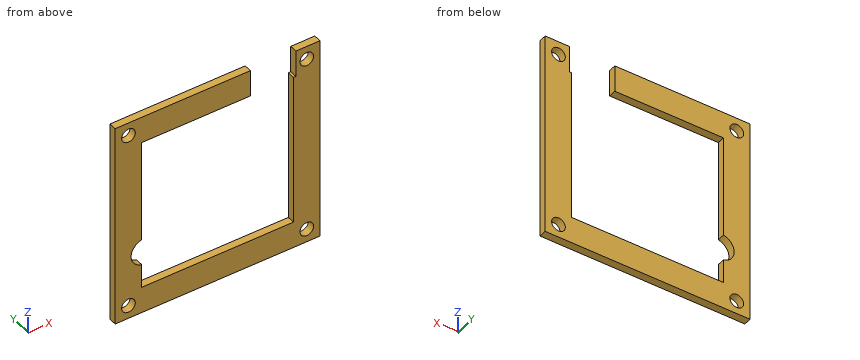
from build123d import *

# Parameters (mm, degrees)
SKETCH_3_R      = 1.8
EXTRUDE_2_DEPTH = 2


with BuildPart() as part:
    # 草图3 → 凸台-拉伸2 (new body)
    with BuildSketch(Plane(origin=(0, 0, 0), x_dir=(1, 0, 0), z_dir=(0, 1, 0))):
        with BuildLine():
            Line((20, 20), (20, -20))
            Line((20, -20), (20.65, -20))
            Line((20.65, -20), (20.65, -27))
            Line((20.65, -27), (27, -27))
            Line((27, -27), (27, 27))
            Line((27, 27), (-27, 27))
            Line((-27, 27), (-27, -27))
            Line((-27, -27), (8.65, -27))
            Line((8.65, -27), (8.65, -20))
            Line((8.65, -20), (-20, -20))
            Line((-20, -20), (-20, 6.87071436))
            ThreePointArc((-20, 6.87071436), (-22.8, 10.3), (-20, 13.72928564))
            Line((-20, 13.72928564), (-20, 20))
            Line((-20, 20), (-16.7, 20))
            Line((-16.7, 20), (-10.4, 20))
            Line((-10.4, 20), (-4.1, 20))
            Line((-4.1, 20), (20, 20))
        make_face()
        with Locations((-23.5, -23.5)):
            Circle(SKETCH_3_R, mode=Mode.SUBTRACT)
        with Locations((23.5, -23.5)):
            Circle(SKETCH_3_R, mode=Mode.SUBTRACT)
        with Locations((-23.5, 23.5)):
            Circle(SKETCH_3_R, mode=Mode.SUBTRACT)
        with Locations((23.5, 23.5)):
            Circle(SKETCH_3_R, mode=Mode.SUBTRACT)
    extrude(amount=EXTRUDE_2_DEPTH)


solid = part.part
Work out the finished part from the listing and answer in its coordinate system (mm). Round coordinates to 2 decimals unless told otherwise and drop trailing zeros. Loops run counter-clockwise (first coordinate to the right, second up) from the corner with the lowest first, then second, coordinate; pieces in that order, holes last. Notation, with made-up numbers: (-14, 54) - (29, 54) arc R13 cw to (29, 71) - close; hole circle Ø9 at (-8, 7). An arc over 180 degrees is marked (long way). One line per item, written item: value.
Q1. Find section B-B on x = 23.5. Give the vertices of the cut face in (y, z).
Check values:
outline: (0, -27) - (2, -27) - (2, -25.3) - (0, -25.3) - close; (0, -21.7) - (2, -21.7) - (2, 21.7) - (0, 21.7) - close; (0, 25.3) - (2, 25.3) - (2, 27) - (0, 27) - close
Q2. Each of these flat-tipped pins is pushed along its axis until it touches: pin 1 Ø0.7 at (x, y) = (20, 0.5) entering from +Z; pin 2 Ø4 at (x, z) = (-23.5, 23.5) entering from +Y; pin 3 Ø3 at (x, z) = (23.5, -23.5) entering from +Y. Where does it stop, or does it pass through?
Check values:
pin 1: z = 20
pin 2: y = 2
pin 3: through
Q3. Find section A-A on z = 6.5. Give the vertices of the cut face in (x, y).
Check values:
outline: (-27, 0) - (-20, 0) - (-20, 2) - (-27, 2) - close; (20, 0) - (27, 0) - (27, 2) - (20, 2) - close
Q4. Straight lines are drawn through the part: probe 1 along X at (y, z) = (0.55, -23.5); probe 2 along X at (y, z) = (1.6, 23.5). For each, find the intervals that lie inside material, in ascending order.
Check values:
probe 1: -27 to -25.3, -21.7 to 21.7, 25.3 to 27
probe 2: -27 to -25.3, -21.7 to 8.65, 20.65 to 21.7, 25.3 to 27
Q5. Find section C-C on y = 0.6. Give the vertices of the cut face in (x, z).
Check values:
outline: (-27, -27) - (27, -27) - (27, 27) - (20.65, 27) - (20.65, 20) - (20, 20) - (20, -20) - (-20, -20) - (-20, -13.73) arc R3.5 cw to (-20, -6.87) - (-20, 20) - (8.65, 20) - (8.65, 27) - (-27, 27) - close; hole circle Ø3.6 at (-23.5, -23.5); hole circle Ø3.6 at (-23.5, 23.5); hole circle Ø3.6 at (23.5, -23.5); hole circle Ø3.6 at (23.5, 23.5)
Q6. Find section D-D on z = 23.5. Give the vertices of the cut face in (x, y).
Check values:
outline: (-27, 0) - (-25.3, 0) - (-25.3, 2) - (-27, 2) - close; (-21.7, 0) - (8.65, 0) - (8.65, 2) - (-21.7, 2) - close; (20.65, 0) - (21.7, 0) - (21.7, 2) - (20.65, 2) - close; (25.3, 0) - (27, 0) - (27, 2) - (25.3, 2) - close
